```python
from build123d import *
from build123d.topology import SkipClean

# Parameters (mm, degrees)
SKETCH2_R               = 3.175
SKETCH2_R_2             = 0.9
BOSS_EXTRUDE1_DEPTH     = 6.35
CUT_EXTRUDE1_DEPTH      = 6.35
FILLET1_R               = 2.54
FILLET2_START           = -7.200738553
FILLET2_DEPTH           = 0.850738553
FILLET2_START_2         = -12.7000001
FILLET2_2_DEPTH         = 5.499261547
CUT_EXTRUDE2_DEPTH      = 74.162913344
CUT_EXTRUDE2_DEPTH_BACK = 74.162913344
SKETCH4_W               = 34.925
SKETCH4_H               = 69.85


with BuildPart() as part:
    # Sketch1 → Revolve1 (revolve)
    with BuildSketch(Plane.XY, mode=Mode.PRIVATE) as revolve1_sk:
        Polygon((0, -50.8), (-31.75, -50.8), (-31.75, 0), (-34.925, 0), (-34.925, -53.975), (0, -53.975), align=None)
    revolve(revolve1_sk.sketch.rotate(Axis((0, -53.975, 0), (0, 1, 0)), 180), axis=Axis((0, -53.975, 0), (0, 1, 0)))

    # Sketch2 → Boss-Extrude1 (add)
    with BuildSketch(Plane(origin=(0, 0, 0), x_dir=(1, 0, 0), z_dir=(0, 1, 0))):
        with Locations((-31.75, 0)):
            Circle(SKETCH2_R)
        with Locations((-31.75, 0)):
            Circle(SKETCH2_R_2, mode=Mode.SUBTRACT)
    extrude(amount=-BOSS_EXTRUDE1_DEPTH)

    # Sketch3 → Cut-Extrude1 (cut)
    with BuildSketch(Plane(origin=(0, 0, 0), x_dir=(1, 0, 0), z_dir=(0, 1, 0))):
        with BuildLine():
            ThreePointArc((-31.737244094, -0.899909599), (-30.85, 0), (-31.737244094, 0.899909599))
            ThreePointArc((-31.737244094, 0.899909599), (-32.65, 0), (-31.737244094, -0.899909599))
        make_face()
    extrude(amount=-CUT_EXTRUDE1_DEPTH, mode=Mode.SUBTRACT)

    # Fillet1
    fillet1_edges = [part.edges().sort_by_distance(p)[0] for p in [
        (-31.59125, -3.175, -3.171028766),
        (-31.59125, -3.175, 3.171028766),
    ]]
    fillet(fillet1_edges, radius=FILLET1_R)

    # Fillet2: read off the stored shape, not the designer's step
    # Fillet2 outline → Fillet2 (add)
    with BuildSketch(Plane(origin=(0, 0, 0), x_dir=(1, 0, 0), z_dir=(0, 1, 0)).offset(FILLET2_START)):
        with BuildLine():
            ThreePointArc((-31.737244094, 0.899909599), (-30.85, 0), (-31.737244094, -0.899909599))
            ThreePointArc((-31.737244094, -0.899909599), (-31.59663833, -3.116880855), (-31.301358696, -5.318594157))
            ThreePointArc((-31.301358696, -5.318594157), (-31.106269167, -3.834791697), (-30.109583333, -2.718392569))
            ThreePointArc((-30.109583333, -2.718392569), (-28.575, 0), (-30.109583333, 2.718392569))
            ThreePointArc((-30.109583333, 2.718392569), (-31.106269167, 3.834791697), (-31.301358696, 5.318594157))
            ThreePointArc((-31.301358696, 5.318594157), (-31.59663833, 3.116880855), (-31.737244094, 0.899909599))
        make_face()
    extrude(amount=FILLET2_DEPTH)

    # Fillet2 2 outline → Fillet2 2 (add)
    with BuildSketch(Plane(origin=(0, 0, 0), x_dir=(1, 0, 0), z_dir=(0, 1, 0)).offset(FILLET2_START_2)):
        with BuildLine():
            ThreePointArc((-31.737244094, 0.899909599), (-30.85, 0), (-31.737244094, -0.899909599))
            ThreePointArc((-31.737244094, -0.899909599), (-31.59663833, -3.116880855), (-31.301358695, -5.318594158))
            ThreePointArc((-31.301358695, -5.318594158), (-31.106269167, -3.834791697), (-30.109583333, -2.718392569))
            ThreePointArc((-30.109583333, -2.718392569), (-28.575, 0), (-30.109583333, 2.718392569))
            ThreePointArc((-30.109583333, 2.718392569), (-31.106269167, 3.834791697), (-31.301358696, 5.318594157))
            ThreePointArc((-31.301358696, 5.318594157), (-31.59663833, 3.116880854), (-31.737244094, 0.899909599))
        make_face()
    extrude(amount=FILLET2_2_DEPTH)

    # Fillet2 3 outline → Fillet2 3 (revolve, cut)
    with BuildSketch(Plane.XY):
        with BuildLine():
            Line((28.575, -12.7000001), (31.75, -12.7))
            ThreePointArc((31.75, -12.7), (30.899261314, -9.525), (28.575, -7.200738685))
            Line((28.575, -7.200738685), (28.575, -12.7000001))
        make_face()
    revolve(axis=Axis((0, 0, 0), (0, 1, 0)), mode=Mode.SUBTRACT)

    # Sketch4 → Cut-Extrude2 (cut, two sides: drawn at the far end of the back side and taken through both)
    with BuildSketch(Plane(origin=(0, 0, 0), x_dir=(1, 0, 0), z_dir=(0, 1, 0)).offset(-CUT_EXTRUDE2_DEPTH_BACK)):
        with Locations((17.4625, 0)):
            Rectangle(SKETCH4_W, SKETCH4_H)
    extrude(amount=CUT_EXTRUDE2_DEPTH + CUT_EXTRUDE2_DEPTH_BACK, mode=Mode.SUBTRACT)

    # Mirror1: part across plane


with BuildPart() as part_1:
    with SkipClean():  # the faces are left unmerged after this step: merging them gives an invalid solid
        add(part.part)
        add(part.part.mirror(Plane(origin=(0, -53.975, 34.925), x_dir=(0, 0, 1), z_dir=(-1, 0, 0))))


solid = part_1.part
```
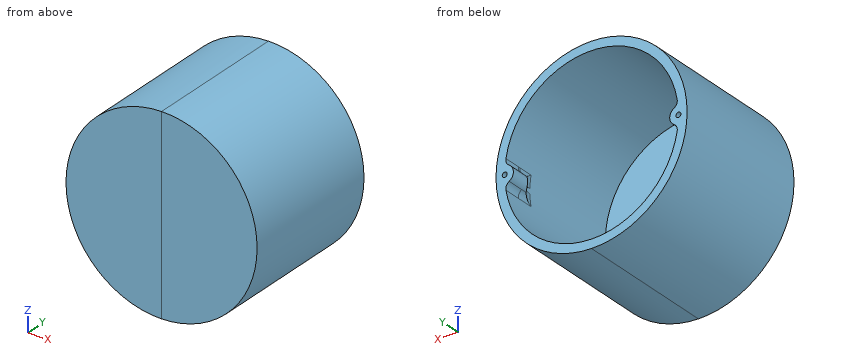
CAD build for the part. Positions are in the model's coordinates, mm. Coordinates: 2 decimals unless noted, no trailing zeros. Order: outer loops, then holes, each group sorted by start corner. A loop starts at its lowest first (then second) coordinate and runs counter-clockwise, first axis right, second up. Notation, with made-up numbers: M -30,-27.75 L 9,-27.75 A20 cw 9,-21.75 Z; hole C -1.75,70 d1. An arc over 180 degrees is marked long. Answer as CSV lines item,"result".
1) Cut at C-C (z = 28). List the corners of the cut face in (x, y) (3 decimals), then the cut area to 3 significant figures.
Verdict:
outline,"M -20.875,-53.975 L 20.875,-53.975 L 20.875,0 L 14.969,0 L 14.969,-50.8 L -14.969,-50.8 L -14.969,0 L -20.875,0 Z"
area,"733 mm2"
2) Cut at A-A (y = -28.5). List the corners of the cut face in (x, z) (3 decimals).
Verdict:
outline,"C 0,0 d69.85; hole C 0,0 d63.5"
3) Cut at D-D (y = -3.5). Give the number of separate pieces and of enclosed holes in the cut face, then the cut area to 3 significant figures.
Verdict:
separate pieces,"1"
enclosed holes,"3"
area,"694 mm2"
4) Cut at B-B (x = 3). List the corners of the cut face in (y, z) (3 decimals), then the cut area to 3 significant figures.
Verdict:
outline,"M -53.975,-34.796 L 0,-34.796 L 0,-31.608 L -50.8,-31.608 L -50.8,31.608 L 0,31.608 L 0,34.796 L -53.975,34.796 Z"
area,"545 mm2"
5) Flat gauge pins, fed straight in: P1, Ø6, axis at x = 11, z = 28, coming from the +Y side; P2, Ø6, axis at x = -26.5, y = -10, coming from the -Z side; P3, Ø1, axis at x = -13, z = -27, coming from the +Y side; P4, Ø1.6, axis at x = -31.75, z = 0, coming from the +Y side. Where does each tip first touch, or does it go through?
Verdict:
P1,"y = 0"
P2,"z = -25.84"
P3,"y = -50.8"
P4,"y = -6.35"
6) Drill centre lines: L1, parallel to Z at x = 1, y = -35; L2, parallel to X at y = -27.5, z = 0 (3 decimals); L3, parallel to Y at x = 9, z = -28.5 (3 decimals). Where is each one in solid material? Low to high. Write a range as from..to.
Verdict:
L1,"-34.91..-31.73, 31.73..34.91"
L2,"-34.925..-31.75, 31.75..34.925"
L3,"-53.975..-50.8"
